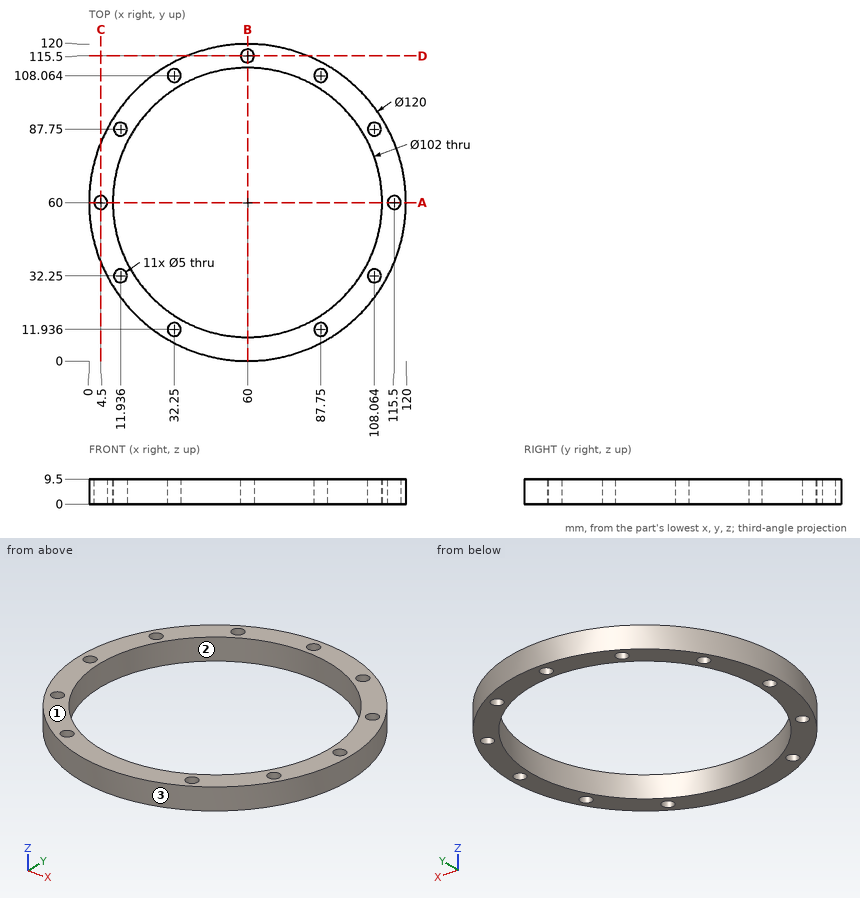
Source: three-view drawing plus pictorial views. Frame: mm from the lowest corner of the part. Coordinates: 2 decimals unless noted, no trailing zeros. Write each loop counter-clockwise with the first axis right and the second up, starting at its lowest first coordinate (ties: lowest second). Pieces come first, ordered by that corner, then holes. Notation, with made-up numbers: (62, 32.5) - (97, 32.5) arc R23 cw to (97, 44.5) - close; hole circle Ø3 at (-12, 31.25). An arc over 180 degrees is marked (long way). Return JSON: item names as keys, results as strings.
Item 1: Line query: L1, parallel to Y at x = 60, z = 2.5; L2, parallel to X at y = 87.75, z = 4.5 (1 decimal); L3, parallel to Y at x = 32, z = 9.25 (1 decimal). Output: solid intervals per line, ascending.
Completed:
{"L1": "y = 0 to 9, 111 to 113, 118 to 120", "L2": "x = 6.8 to 9.4, 14.4 to 17.2, 102.8 to 105.6, 110.6 to 113.2", "L3": "y = 6.9 to 9.4, 14.4 to 17.4, 102.6 to 105.6, 110.6 to 113.1"}
Item 2: Section query B-B (x = 60). Output: boundary loops of the cut face in (y, z).
Completed:
{"outline": "(0, 0) - (9, 0) - (9, 9.5) - (0, 9.5) - close; (111, 0) - (113, 0) - (113, 9.5) - (111, 9.5) - close; (118, 0) - (120, 0) - (120, 9.5) - (118, 9.5) - close"}
Item 3: Pull-direction query (Y, two-part tool) for the marked faces 1, 2 and 3; classes: +Y half, -Y half, draft (parallel to the pull), parting line (faces both ways), or undercut.
Completed:
{"face 1": "draft", "face 2": "undercut", "face 3": "parting line"}
Item 4: Section query C-C (x = 4.5). Output: boundary loops of the cut face in (y, z), and give its area (3 significant figures).
Completed:
{"outline": "(37.2, 0) - (57.5, 0) - (57.5, 9.5) - (37.2, 9.5) - close; (62.5, 0) - (82.8, 0) - (82.8, 9.5) - (62.5, 9.5) - close", "area": "386 mm2"}
Item 5: Pin query (flat end, axial travel): pin 1 Ø4 at (x, y) = (11.94, 87.75) entering from +Z; pin 2 Ø5 at (y, z) = (21, 1.5) entering from -X; pin 3 Ø2 at (x, z) = (71.5, 3) entering from +Y; pin 4 Ø1 at (y, z) = (52.5, 2) entering from -X. Return the tip coordinate at first contact, or that it passes through.
Completed:
{"pin 1": "passes through", "pin 2": "stops at x = 12.38", "pin 3": "stops at y = 119.07", "pin 4": "stops at x = 0.41"}
Item 6: Section query A-A (y = 60). Output: boundary loops of the cut face in (x, z).
Completed:
{"outline": "(0, 0) - (2, 0) - (2, 9.5) - (0, 9.5) - close; (7, 0) - (9, 0) - (9, 9.5) - (7, 9.5) - close; (111, 0) - (113, 0) - (113, 9.5) - (111, 9.5) - close; (118, 0) - (120, 0) - (120, 9.5) - (118, 9.5) - close"}
